The listing builds one solid part. Answer for the finished solid, in the listing's coordinates (mm). Face numbers are marked on the shaded views. A direction names the side the tool comes from. Round coordinates to 2 decimals unless told otherwise and drop trailing zeros. Write each loop counter-clockwise with the first axis right and the second up, starting at its lowest first coordinate (ties: lowest second). Pieces come first, ordered by that corner, then holes. Notation, with made-up numbers: M 54.25,16.5 L 99.25,16.5 A12 cw 99.25,22.5 Z; hole C 38,-27.5 d4. An arc over 180 degrees is marked long. Answer as CSV lines item,"result". Start each with the question number.
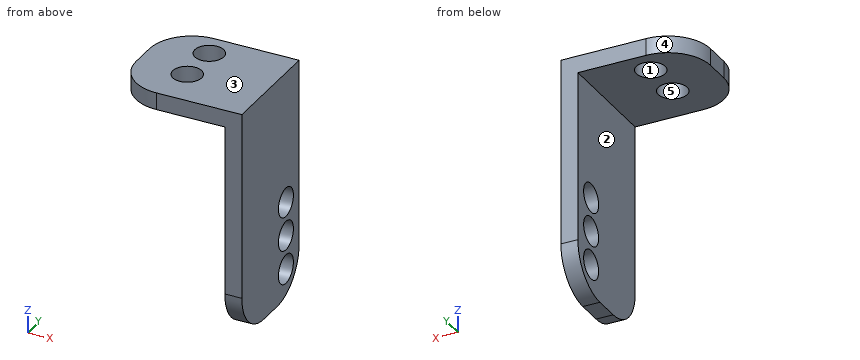
from build123d import *

# Parameters (mm, degrees)
F0_W     = 2
F0_H     = 20
F0_W_2   = 13
F1_DEPTH = 2
F2_D     = 3.4
F3_DEPTH = 25
F5_D     = 3.4
F6_DEPTH = 7
F7_R     = 5


with BuildPart() as f1:
    # F0 (on Top) → F1 (new body)
    with BuildSketch(Plane.XY):
        with Locations((6.5, 0)):
            Rectangle(F0_W, F0_H)
        with Locations((-1, 0)):
            Rectangle(F0_W_2, F0_H)
    extrude(amount=F1_DEPTH)

    # F2 (through all)
    with Locations(Plane(origin=(0, 0, 0), x_dir=(1, 0, 0), z_dir=(0, 0, -1))):
        with Locations((-1.5, -5), (-1.5, 0), (-1.5, 5)):
            Hole(F2_D / 2)

    # F0 (on Top) → F3 (join)
    with BuildSketch(Plane.XY):
        with Locations((6.5, 0)):
            Rectangle(F0_W, F0_H)
    extrude(amount=-F3_DEPTH)

    # F5 (through all)
    with Locations(Plane(origin=(5.5, 0, 0), x_dir=(0, -1, 0), z_dir=(-1, 0, 0))):
        with Locations((0, -17.5), (0, -13.5), (0, -21.5)):
            Hole(F5_D / 2)

    # F6 (cut): a face of the model
    f6_faces = [f1.faces().sort_by_distance(p)[0] for p in [
        (0, 10, 1.6911310958),
    ]]
    extrude(f6_faces, amount=-F6_DEPTH, mode=Mode.SUBTRACT)

    # F7
    f7_edges = [f1.edges().sort_by_distance(p)[0] for p in [
        (6.5, 3, -25),
        (6.5, -10, -25),
        (-7.5, -10, 1),
        (-7.5, 3, 1),
    ]]
    fillet(f7_edges, radius=F7_R)


solid = f1.part
Q1. Find section D-D (z = -12.5). Determine the outline of the cut face in (x, y).
Q2. Find section C-C (y = 0). Determine the outline of the cut face in (x, z), plus the area to 3 significant figures.
Q3. For the marked faces 1 and 2, determine the directions among +Z, -Z, +X, -X, +Y, -Y from which every point of the face is accessible in a straight line to the end or side of a thin tool.
Q4. Find section A-A (z = -17.5). Determine the outline of the cut face in (x, y).
Q5. Find section B-B (y = -4). Determine the outline of the cut face in (x, z).
Q6. The mould has two halves that part along X. Classify the marked faces 3, 4 and 5: +X half, -X half, draft (parallel to the pull), parting line (faces both ways), or undercut.
Q7. Straight lines are drawn through the part: L1, parallel to Y at x = -1.5, z = 1.3; L2, parallel to Z at x = 5.9, y = 0; L3, parallel to Y at x = -0.25, z = 0.25. For each, find the intervals that lie inside material, in ascending order.
Q8. Each of these flat-tipped pins is pushed along its axis until it touches: P1, Ø1, axis at y = -4, z = -3, coming from the -X side; P2, Ø1.5, axis at x = -1, y = -4, coming from the +Z side; P3, Ø6.5, axis at x = -1, y = -2.5, coming from the -Z side. Where does it stop, or does it pass through?
Reported:
1,outline,"M 5.5,-10 L 7.5,-10 L 7.5,-1.37 L 5.5,-1.37 Z; M 5.5,1.37 L 7.5,1.37 L 7.5,3 L 5.5,3 Z"
2,outline,"M -7.08,0 L -3.2,0 L -3.2,2 L -7.08,2 Z; M 0.2,0 L 5.5,0 L 5.5,-11.8 L 7.5,-11.8 L 7.5,2 L 0.2,2 Z; M 5.5,-24.58 L 7.5,-24.58 L 7.5,-23.2 L 5.5,-23.2 Z; M 5.5,-19.8 L 7.5,-19.8 L 7.5,-19.2 L 5.5,-19.2 Z; M 5.5,-15.8 L 7.5,-15.8 L 7.5,-15.2 L 5.5,-15.2 Z"
2,area,"51.1 mm2"
3,face 1,"+Z, -Z"
3,face 2,"-Z, -X, +Y, -Y"
4,outline,"M 5.5,-10 L 7.5,-10 L 7.5,-1.7 L 5.5,-1.7 Z; M 5.5,1.7 L 7.5,1.7 L 7.5,3 L 5.5,3 Z"
5,outline,"M -7.5,0 L -2.87,0 L -2.87,2 L -7.5,2 Z; M -0.13,0 L 5.5,0 L 5.5,-25 L 7.5,-25 L 7.5,2 L -0.13,2 Z"
6,face 3,"draft"
6,face 4,"-X half"
6,face 5,"undercut"
7,L1,"y = -10 to -6.7, -3.3 to -1.7, 1.7 to 3"
7,L2,"z = -24.58 to -23.2, -19.8 to -19.2, -15.8 to -15.2, -11.8 to 2"
7,L3,"y = -10 to -6.15, -3.85 to -1.15, 1.15 to 3"
8,P1,"stops at x = 5.5"
8,P2,"stops at z = 2"
8,P3,"stops at z = 0"
